from build123d import *

# Parameters (mm, degrees)
SKETCH1_W           = 70
SKETCH1_H           = 13
BOSS_EXTRUDE1_DEPTH = 5
CUT_EXTRUDE1_DEPTH  = 36.947878936
BOSS_EXTRUDE3_START = 5
SKETCH2_3_W         = 18.390349325
SKETCH2_3_H         = 13
SKETCH2_3_R         = 2
BOSS_EXTRUDE3_DEPTH = 5
SKETCH3_R           = 2.5
BOSS_EXTRUDE4_DEPTH = 10


with BuildPart() as part:
    # Sketch1 → Boss-Extrude1 (new body)
    with BuildSketch(Plane(origin=(0, 0, 0), x_dir=(1, 0, 0), z_dir=(0, 1, 0))):
        Rectangle(SKETCH1_W, SKETCH1_H)
    extrude(amount=BOSS_EXTRUDE1_DEPTH)

    # Sketch2 → Cut-Extrude1 (cut, through all)
    with BuildSketch(Plane(origin=(0, 5, 0), x_dir=(1, 0, 0), z_dir=(0, 1, 0))):
        with BuildLine():
            ThreePointArc((-22.141309667, 0), (-24.141309667, 2), (-26.141309667, 0))
            Line((-26.141309667, 0), (-22.141309667, 0))
        make_face()
        with BuildLine():
            Line((-22.141309667, 0), (-26.141309667, 0))
            ThreePointArc((-26.141309667, 0), (-24.141309667, -2), (-22.141309667, 0))
        make_face()
        with BuildLine():
            ThreePointArc((-12.141309667, 0), (-14.141309667, 2), (-16.141309667, 0))
            Line((-16.141309667, 0), (-12.141309667, 0))
        make_face()
        with BuildLine():
            Line((-12.141309667, 0), (-16.141309667, 0))
            ThreePointArc((-16.141309667, 0), (-14.141309667, -2), (-12.141309667, 0))
        make_face()
    extrude(amount=-CUT_EXTRUDE1_DEPTH, mode=Mode.SUBTRACT)

    # Sketch2_3 → Boss-Extrude3 (add)
    with BuildSketch(Plane(origin=(0, 5, 0), x_dir=(1, 0, 0), z_dir=(0, 1, 0)).offset(BOSS_EXTRUDE3_START)):
        with Locations((-19.114378827, 0)):
            Rectangle(SKETCH2_3_W, SKETCH2_3_H)
        with Locations(Location((-24.141309667, 0, 0), (0, 0, 270))):
            Circle(SKETCH2_3_R, mode=Mode.SUBTRACT)
        with Locations(Location((-14.141309667, 0, 0), (0, 0, 270))):
            Circle(SKETCH2_3_R, mode=Mode.SUBTRACT)
    extrude(amount=-BOSS_EXTRUDE3_DEPTH)

    # Sketch3 → Boss-Extrude4 (add)
    with BuildSketch(Plane(origin=(0, 0, 0), x_dir=(-1, 0, 0), z_dir=(0, -1, 0))):
        with Locations(Location((-13.394545769, 0, 0), (0, 0, 270))):
            Circle(SKETCH3_R)
    extrude(amount=BOSS_EXTRUDE4_DEPTH)


solid = part.part
Work out the finished part from the listing and answer in its coordinate system (mm). A direction names the side the tool comes from. Give positions to 0.01 mm unless a question says otherwise; leave off trailing zeros. Loops run counter-clockwise (first coordinate to the right, second up) from the corner with the lowest first, then second, coordinate; pieces in that order, holes last. Notation, with made-up numbers: (-5.5, 77) - (1.5, 77) arc R21 ccw to (1.5, 87) - close; hole circle Ø7 at (-30.75, 77.5). An arc over 180 degrees is marked (long way). Answer in a Markdown table with one row per item. Add a question column.
Q1. The part is cut by section C-C (x = 15). Determine the outline of the cut face in (y, z).
Q2. The part is cut by section B-B (y = 2.5). Determine the outline of the cut face in (x, z).
Q3. The part is cut by section D-D (y = -4.25). Determine the outline of the cut face in (x, z).
Q4. Consider line 1 along X through (y, z) = (6.5, 0); line 2 along X through (y, z) = (4.75, 0); line 3 along Y through (x, z) = (0, 5.75). Determine where each line is inside the solid, lowest interval first.
Q5. Each of these flat-tipped pins is pushed along its axis until it touches: P1, Ø4, axis at y = -5.5, z = -4, coming from the -X side; P2, Ø6.5, axis at x = -24.14, z = 0, coming from the +Y side; P3, Ø2, axis at x = 16, z = -4, coming from the -Y side; P4, Ø1, axis at x = 15, y = -3.5, coming from the +Z side. Where does it stop, or does it pass through?
Q6. The part is cut by section A-A (z = -5). Determine the outline of the cut face in (x, y).
Q7. Determine the mould class of faces 6 (the cylindrical face through (-15.71, 5.07, -1.24)), 7 (the flat face through (-8, 3, 6.5)), 8 (the flat face through (-9.919, 8, 0)) for opening direction Z: released by +Z, released by -Z, zero draft, split by the parting line, or undercut.
Q8. A tool of negligible diameter and unlimited length cuts with its end or side. For faces 1 (the cylindrical face through (15.835, -4.93, -0.542)), 2 (the flat face through (-32, 5, 0)), 3 (the flat face through (-19, 10, 0)), 4 (the flat face through (-35, 2, 0)), 5 (the flat face through (12, 5, 0)), from which of +Z, -Z, +X, -X, +Y, -Y can it reach the whole face along a straight path? Write none if from no direction.
Solution:
| question | item | result |
|---|---|---|
| 1 | outline | (-10, -1.92) - (0, -1.92) - (0, -6.5) - (5, -6.5) - (5, 6.5) - (0, 6.5) - (0, 1.92) - (-10, 1.92) - close |
| 2 | outline | (-35, -6.5) - (35, -6.5) - (35, 6.5) - (-35, 6.5) - close; hole circle Ø4 at (-24.14, 0); hole circle Ø4 at (-14.14, 0) |
| 3 | outline | circle Ø5 at (13.39, 0) |
| 4 | line 1 | x = -28.31 to -26.14, -22.14 to -16.14, -12.14 to -9.92 |
| 4 | line 2 | x = -35 to -26.14, -22.14 to -16.14, -12.14 to 35 |
| 4 | line 3 | y = 0 to 5 |
| 5 | P1 | stops at x = 11.89 |
| 5 | P2 | stops at y = 10 |
| 5 | P3 | stops at y = 0 |
| 5 | P4 | stops at z = 2.24 |
| 6 | outline | (-35, 0) - (35, 0) - (35, 5) - (-9.92, 5) - (-9.92, 10) - (-28.31, 10) - (-28.31, 5) - (-35, 5) - close |
| 7 | face 6 | undercut |
| 7 | face 7 | released by +Z |
| 7 | face 8 | zero draft |
| 8 | face 1 | -Y |
| 8 | face 2 | +Z, -Z, -X, +Y |
| 8 | face 3 | +Z, -Z, +X, -X, +Y |
| 8 | face 4 | +Z, -Z, -X, +Y, -Y |
| 8 | face 5 | +Z, -Z, +X, +Y |
